Autodesk Inventor part; units mm, degrees
ref_plane "YZ Plane" through (0, 0, 0) normal (1, 0, 0) x (0, 1, 0)
ref_plane "XZ Plane" through (0, 0, 0) normal (0, 1, 0) x (-1, 0, 0)
ref_plane "XY Plane" through (0, 0, 0) normal (0, 0, 1) x (1, 0, 0)
sketch "Sketch1" plane through (0, 0, 0) normal (0, 1, 0) x (-1, 0, 0)
  line L0 (37.5811, -104.7549) -> (37.5811, -130.1549)
  line L1 (62.9811, -155.5549) -> (164.5811, -155.5549)
  line L2 (189.9811, -130.1549) -> (189.9811, -104.7549)
  arc A0 (62.9811, -155.5549) -> (37.5811, -130.1549) centre (50.2811, -142.8549) ccw
  arc A1 (189.9811, -130.1549) -> (164.5811, -155.5549) centre (177.2811, -142.8549) ccw
  arc A2 (164.5811, -79.3549) -> (189.9811, -104.7549) centre (177.2811, -92.0549) ccw
  arc A3 (37.5811, -104.7549) -> (62.9811, -79.3549) centre (50.2811, -92.0549) ccw
  line L3 (164.5811, -79.3549) -> (62.9811, -79.3549)
  point P0 (0, 0)
  dimension "d4" = 17.9605
  dimension "d11" = 17.9605
  dimension "d16" = 25.4
  dimension "d17" = 17.9605
  dimension "d18" = 25.4
  dimension "d19" = 101.6
  dimension "d20" = 17.9605
extrude "Extrusion1" add sketch "Sketch1" along normal blind 1.5875
sketch "Sketch2" plane through (0, 1.5875, 0) normal (0, 1, 0) x (1, 0, 0)
  circle A0 centre (-113.7811, 117.4549) radius 2.7481
  line L0 (-62.9811, 155.5549) -> (-164.5811, 155.5549)
  line L1 (-37.5811, 104.7549) -> (-37.5811, 130.1549)
  circle A1 centre (-145.5311, 117.4549) radius 2.7481
  circle A2 centre (-177.2811, 117.4549) radius 2.7481
  circle A3 centre (-82.0311, 117.4549) radius 2.7481
  circle A4 centre (-50.2811, 117.4549) radius 2.7481
  circle A5 centre (-113.7811, 142.8549) radius 2.7481
  circle A6 centre (-113.7811, 92.0549) radius 2.7481
  point P0 (0, 0)
  dimension "d23" = 38.1
  dimension "d24" = 76.2
  dimension "d27" = 31.75
  dimension "d34" = 31.75
  dimension "d41" = 25.4
  dimension "d48" = 25.4
extrude "Extrusion2" add sketch "Sketch2" along normal blind 0.508
sketch "Sketch3" plane through (-189.9811, 0, -130.1549) normal (-1, 0, 0) x (0, 0, 1)
  line L0 (24.5513, 1.3891) -> (4.2313, 1.3891)
  line L1 (4.2313, 1.3891) -> (4.2313, 0.1984)
  line L2 (4.2313, 0.1984) -> (24.5513, 0.1984)
  line L3 (24.5513, 0.1984) -> (24.5513, 1.3891)
  line L4 (0, 0) -> (0, 1.5875)
  line L5 (0, 0) -> (25.4, 0)
  line L6 (25.4, 0) -> (25.4, 1.5875)
  line L7 (0, 1.5875) -> (25.4, 1.5875)
  point P0 (130.1549, 0)
  dimension "d55" = 1.5875
  dimension "d56" = 25.4
  dimension "d57" = 1.1906
  dimension "d58" = 0.1984
  dimension "d59" = 20.32
sketch "Sketch4" plane through (-37.5811, 0, -104.7549) normal (1, 0, 0) x (0, 0, -1)
  line L0 (0, 1.5875) -> (25.4, 1.5875)
  line L1 (0, 0) -> (0, 1.5875)
  line L2 (25.4, 0) -> (25.4, 1.5875)
  line L3 (0.9323, 0.1905) -> (21.2523, 0.1905)
  line L4 (21.2523, 0.1905) -> (21.2523, 1.3843)
  line L5 (21.2523, 1.3843) -> (0.9323, 1.3843)
  line L6 (0.9323, 1.3843) -> (0.9323, 0.1905)
  point P0 (-104.7549, 0)
  dimension "d60" = 20.32
  dimension "d61" = 1.1938
  dimension "d62" = 0.2032
extrude "Extrusion3" add sketch "Sketch4" along normal blind 0.508
sketch "Sketch5" plane through (-62.9811, 0, -155.5549) normal (0, 0, -1) x (-1, 0, 0)
  line L0 (101.6, 0) -> (101.6, 1.5875)
  line L1 (0, 0) -> (0, 1.5875)
  line L2 (40.64, 0.2032) -> (60.96, 0.2032)
  line L3 (60.96, 0.2032) -> (60.96, 1.397)
  line L4 (60.96, 1.397) -> (40.64, 1.397)
  line L5 (40.64, 1.397) -> (40.64, 0.2032)
  line L6 (0, 1.5875) -> (101.6, 1.5875)
  line L7 (0, 0) -> (101.6, 0)
  point P0 (-62.9811, 0)
  dimension "d65" = 20.32
  dimension "d66" = 40.64
  dimension "d67" = 101.6
  dimension "d68" = 40.64
  dimension "d69" = 1.1938
  dimension "d70" = 0.2032
  dimension "d71" = 0.1905
extrude "Extrusion4" add sketch "Sketch5" along normal blind 0.508 contours L5 L4 L3 L2
extrude "Extrusion5" add sketch "Sketch3" along normal blind 0.508 contours L3 L2 L1 L0
sketch "Sketch6" plane through (-164.5811, 0, -79.3549) normal (0, 0, 1) x (1, 0, 0)
  line L0 (101.6, 0) -> (101.6, 1.5875)
  line L1 (0, 0) -> (0, 1.5875)
  line L2 (60.96, 0.2032) -> (40.64, 0.2032)
  line L3 (40.64, 0.2032) -> (40.64, 1.397)
  line L4 (40.64, 1.397) -> (60.96, 1.397)
  line L5 (60.96, 1.397) -> (60.96, 0.2032)
  line L6 (0, 0) -> (101.6, 0)
  point P0 (164.5811, 0)
  dimension "d76" = 20.32
  dimension "d77" = 1.1938
  dimension "d78" = 0.2032
  dimension "d79" = 40.64
extrude "Extrusion6" add sketch "Sketch6" along normal blind 0.508
equation "\"d57\" = 0.75 * d55"
equation "\"d58\" = -0.5 * d57 + 0.5 * d55"
properties part number "FORS phone case- base"
Geometry check sheet. Reference: the model listing, model coordinates, mm. A direction names the side the tool comes from. Round coordinates to 2 decimals unless told otherwise and drop trailing zeros. Loops run counter-clockwise (first coordinate to the right, second up) from the corner with the lowest first, then second, coordinate; pieces in that order, holes last. Notation, with made-up numbers: (68, 57) - (100, 57) arc R6 ccw to (100, 64) - close; hole circle Ø4 at (1, 38.25). An arc over 180 degrees is marked (long way). One line per question, with ' | ' between items. Start each with the question number.
1. Tool access check on faces 4 (the face through (-82, 2.096, -117)), 5 (the face through (-113, 1.588, -125)). Record the directions out of +Z, -Z, +X, -X, +Y, -Y that give a thin tool (end or side, any length) a straight path to the whole face; none if there is none.
2. Cross-section at C-C on z = -128.5. Record the cut outline in (x, y).
3. Draft check along X on faces 1 (the face through (-63.26, 0.78, -104.47)), 2 (the face through (-114, 2.096, -143)), 3 (the face through (-111.16, 1.84, -91.23)). Enter one of: released by +X, released by -X, zero draft, split by the parting line, or undercut.
4. Cross-section at A-A on y = 1.05. Record the cut outline in (x, z), then the cut area to 3 significant figures.
5. Cross-section at B-B on z = -112. Record the cut outline in (x, y), then the cut area to 3 significant figures.
6. Cross-section at D-D on x = -99. Record the cut outline in (y, z), then the cut area to 3 significant figures.
7. Scan lines: line 1 (X direction, y = 0.2, z = -128.5); line 2 (Y direction, x = -180, z = -124); line 3 (Z direction, x = -100.5, y = 0.7). Record each from-to range of solid material in increasing order. Write a range as [from, to].
8. Depth check by flat-ended pin: pin 1 (4 mm diameter, centred on x = -158.5, z = -134.5, fed in from +Y); pin 2 (0.6 mm diameter, centred on y = 0.5, z = -156, fed in from +X); pin 3 (0.6 mm diameter, centred on x = -190.5, z = -115.5, fed in from +Y). Enter the tip coordinate at first touch or a pass-through.
Taken from the geometry:
1) face 4: +Z, -Z, +X, -X, +Y | face 5: +Y
2) outline: (-189.98, 0) - (-188.08, 0) - (-188.08, 1.59) - (-189.98, 1.59) - close; (-166.49, 0) - (-61.08, 0) - (-61.08, 1.59) - (-166.49, 1.59) - close; (-39.49, 0) - (-37.58, 0) - (-37.58, 1.59) - (-39.49, 1.59) - close
3) face 1: undercut | face 2: zero draft | face 3: split by the parting line
4) outline: (-190.49, -125.92) - (-189.98, -125.92) - (-189.98, -130.15) arc R17.96 cw to (-164.58, -155.55) - (-123.94, -155.55) - (-123.94, -156.06) - (-103.62, -156.06) - (-103.62, -155.55) - (-62.98, -155.55) arc R17.96 cw to (-37.58, -130.15) - (-37.58, -126.01) - (-37.07, -126.01) - (-37.07, -105.69) - (-37.58, -105.69) - (-37.58, -104.75) arc R17.96 cw to (-62.98, -79.35) - (-103.62, -79.35) - (-103.62, -78.85) - (-123.94, -78.85) - (-123.94, -79.35) - (-164.58, -79.35) arc R17.96 cw to (-189.98, -104.75) - (-189.98, -105.6) - (-190.49, -105.6) - close | area: 8,340 mm²
5) outline: (-190.49, 0.2) - (-189.98, 0.2) - (-189.98, 0) - (-37.58, 0) - (-37.58, 0.19) - (-37.07, 0.19) - (-37.07, 1.38) - (-37.58, 1.38) - (-37.58, 1.59) - (-189.98, 1.59) - (-189.98, 1.39) - (-190.49, 1.39) - close | area: 243 mm²
6) outline: (0, -155.55) - (1.59, -155.55) - (1.59, -79.35) - (0, -79.35) - close | area: 121 mm²
7) line 1: [-189.98, -188.08], [-166.49, -61.08], [-39.49, -37.58] | line 2: [0, 1.59] | line 3: [-155.55, -79.35]
8) pin 1: y = 1.59 | pin 2: x = -103.62 | pin 3: y = 1.39
